Autodesk Inventor part; units mm, degrees
ref_plane "YZ Plane" through (0, 0, 0) normal (1, 0, 0) x (0, 1, 0)
ref_plane "XZ Plane" through (0, 0, 0) normal (0, 1, 0) x (-1, 0, 0)
ref_plane "XY Plane" through (0, 0, 0) normal (0, 0, 1) x (1, 0, 0)
sketch "Sketch1" plane through (0, 0, 0) normal (0, 0, 1) x (1, 0, 0)
  line L0 (0, 0) -> (300, 0)
  line L1 (300, 0) -> (300, 200)
  line L2 (300, 200) -> (0, 200)
  line L3 (0, 200) -> (0, 0)
  dimension "d0" = 300
  dimension "d1" = 200
extrude "Extrusion1" add sketch "Sketch1" along normal blind 10
sketch "Sketch2" plane through (0, 0, 0) normal (0, 0, -1) x (-1, 0, 0)
  circle A0 centre (-80, 100) radius 50
  line L0 (-300, 200) -> (0, 200)
  line L1 (0, 200) -> (0, 0)
  dimension "d4" = 100
  dimension "d5" = 100
  dimension "d6" = 80
extrude "Extrusion2" cut sketch "Sketch2" against normal through all
sketch "Sketch3" plane through (0, 0, 10) normal (0, 0, 1) x (1, 0, 0)
  point P0 (0, 0)
sketch "Sketch4" plane through (0, 0, 10) normal (0, 0, 1) x (1, 0, 0)
  circle A0 centre (265, 100) radius 5
  line L0 (0, 0) -> (300, 0)
  line L1 (300, 0) -> (300, 200)
  dimension "d9" = 10
  dimension "d10" = 100
  dimension "d11" = 30
extrude "Extrusion3" cut sketch "Sketch4" against normal through all
sketch "Sketch5" plane through (0, 0, 0) normal (0, 0, -1) x (-1, 0, 0)
  circle A0 centre (-6.4515, 6.4515) radius 1.4515
  circle A1 centre (-293.5485, 193.5485) radius 1.4515
  circle A2 centre (-293.5485, 6.4515) radius 1.4515
  line L0 (0, 200) -> (0, 0)
  line L1 (0, 0) -> (-300, 0)
  circle A3 centre (-6.4515, 193.5485) radius 1.4515
  line L2 (-300, 200) -> (0, 200)
  line L3 (-300, 0) -> (-300, 200)
  dimension "d14" = 2.903
  dimension "d16" = 2.903
  dimension "d17" = 2.903
  dimension "d18" = 5
  dimension "d19" = 5
  dimension "d20" = 2.903
  dimension "d21" = 5
  dimension "d22" = 5
  dimension "d23" = 5
  dimension "d24" = 5
  dimension "d25" = 5
  dimension "d26" = 5
extrude "Extrusion4" cut sketch "Sketch5" against normal through all contours A0 | A1 | A2 | A3
equation "\"BendRadius\" = Thickness"
equation "\"BendReliefWidth\" = Thickness"
equation "\"BendReliefDepth\" = 0.5 * Thickness"
equation "\"CornerReliefSize\" = 4 * Thickness"
equation "\"MinimumRemnant\" = 2 * Thickness"
equation "\"TransitionRadius\" = BendRadius"
equation "\"JacobiRadiusSize\" = BendRadius"
equation "\"GapSize\" = Thickness"
properties part number "base cap"
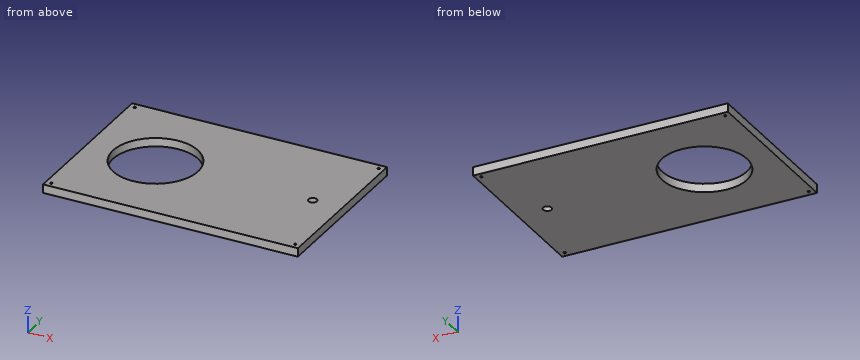
Geometry check sheet. Reference: the model listing, model coordinates, mm. Round coordinates to 2 decimals unless told otherwise and drop trailing zeros. Order: outer loops, then holes, each group sorted by start corner. A loop starts at its lowest first (then second) coordinate and runs counter-clockwise, first axis right, second up. Notation, with made-up numbers: (-17.75, -5.5) - (-5.75, -5.5) arc R37 cw to (-5.75, 32.5) - close; hole circle Ø9 at (36.5, 8). An arc over 180 degrees is marked (long way). Use a Markdown table: item, result. Add a question column.
1) Section check A-A (x = 265). Record the cut outline in (y, z).
2) Section check D-D (z = 2.25). Record the cut outline in (x, y).
3) Section check B-B (y = 100). Record the cut outline in (x, z).
4) Thickness scan on line 1 along Y through (x, z) = (80, 7); line 2 along Y through (x, z) = (101, 8.5); line 3 along X through (y, z) = (85.5, 4.25). Record the ranges inside material, lowest first.
5) Section check C-C (y = 61). Record the cut outline in (x, z).
6) Gauge pin test, flat end, axial feed: P1, Ø13, axis at x = 265, y = 100, coming from the +Z side. Record the tip position at first contact, or that the pin passes through.
Established:
| question | item | result |
|---|---|---|
| 1 | outline | (0, 0) - (95, 0) - (95, 10) - (0, 10) - close; (105, 0) - (200, 0) - (200, 10) - (105, 10) - close |
| 2 | outline | (0, 0) - (300, 0) - (300, 200) - (0, 200) - close; hole circle Ø2.9 at (6.45, 6.45); hole circle Ø2.9 at (6.45, 193.55); hole circle Ø100 at (80, 100); hole circle Ø10 at (265, 100); hole circle Ø2.9 at (293.55, 6.45); hole circle Ø2.9 at (293.55, 193.55) |
| 3 | outline | (0, 0) - (30, 0) - (30, 10) - (0, 10) - close; (130, 0) - (260, 0) - (260, 10) - (130, 10) - close; (270, 0) - (300, 0) - (300, 10) - (270, 10) - close |
| 4 | line 1 | 0 to 50, 150 to 200 |
| 4 | line 2 | 0 to 54.62, 145.38 to 200 |
| 4 | line 3 | 0 to 32.15, 127.85 to 300 |
| 5 | outline | (0, 0) - (48.71, 0) - (48.71, 10) - (0, 10) - close; (111.29, 0) - (300, 0) - (300, 10) - (111.29, 10) - close |
| 6 | P1 | z = 10 |
